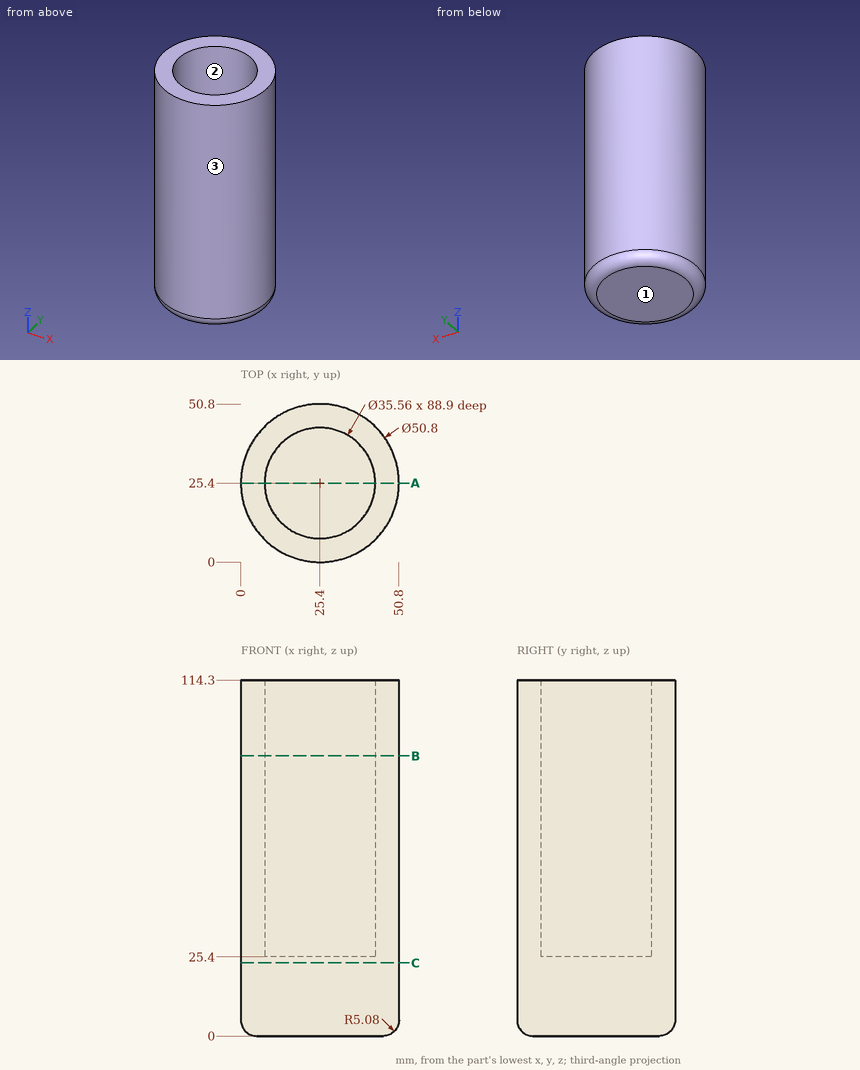
Here's the drawing with two shaded views (mm, measured from the low corner). I have some questions. Give positions to 0.01 mm unless a question says otherwise; leave off trailing zeros. Loops run counter-clockwise (first coordinate to the right, second up) from the corner with the lowest first, then second, coordinate; pieces in that order, holes last. Notation, with made-up numbers: (-17, 44) - (40, 44) arc R30 ccw to (40, 74) - close; hole circle Ø5 at (20.25, -22.5). An arc over 180 degrees is marked (long way). Return JSON: item names as keys, results as strings.
1. We'd pull the mould along X, two halves only. Please class the marked faces 1, 2 and 3: +X half, -X half, draft (parallel to the pull), parting line (faces both ways), or undercut.
Output values:
{"face 1": "draft", "face 2": "undercut", "face 3": "parting line"}
2. I want a section at C-C on z = 23.5. Please give me the cut outline in (x, y), and give its area (3 significant figures).
Output values:
{"outline": "circle Ø50.8 at (25.4, 25.4)", "area": "2,030 mm²"}
3. I want a section at B-B on z = 90. Please give me the cut outline in (x, y), and give its area (3 significant figures).
Output values:
{"outline": "circle Ø50.8 at (25.4, 25.4); hole circle Ø35.56 at (25.4, 25.4)", "area": "1,030 mm²"}
4. If I drill on line 1 (X direction, y = 25, z = 45); line 2 (Z direction, x = 20, y = 35.5); line 3 (Y direction, x = 20.5, z = 50.5), over which ranges is the centre line in solid material (lowest first)?
Output values:
{"line 1": "x = 0 to 7.62, 43.18 to 50.8", "line 2": "z = 0 to 25.4", "line 3": "y = 0.48 to 8.31, 42.49 to 50.32"}
5. I want a section at A-A on y = 25.4. Please give me the cut outline in (x, z).
Output values:
{"outline": "(0, 5.08) arc R5.08 ccw to (5.08, 0) - (45.72, 0) arc R5.08 ccw to (50.8, 5.08) - (50.8, 114.3) - (43.18, 114.3) - (43.18, 25.4) - (7.62, 25.4) - (7.62, 114.3) - (0, 114.3) - close"}
6. I'm going to push flat-ended pins straight in: pin 1 Ø1.5 at (y, z) = (33.5, 48.5) entering from +X; pin 2 Ø1 at (y, z) = (44, 44.5) entering from +X; pin 3 Ø5 at (y, z) = (32, 29.5) entering from +X. Where does each tip first touch, or does it pass through?
Output values:
{"pin 1": "stops at x = 49.71", "pin 2": "stops at x = 43.22", "pin 3": "stops at x = 50.47"}
